from build123d import *

# Parameters (mm, degrees)
ESBO_O1_W                         = 40
ESBO_O1_H                         = 15
RESSALTO_EXTRUS_O1_DEPTH          = 3
ESBO_O3_W                         = 40
ESBO_O3_H                         = 15
RESSALTO_EXTRUS_O2_DEPTH          = 2
CORTE_EXTRUS_O1_REACH             = 26.418
ESBO_O2_R                         = 2.5
ESBO_O2_R_2                       = 0.75
CORTE_EXTRUS_O1_DIRECTION_2_REACH = 26.418
ESBO_O5_W                         = 20
ESBO_O5_H                         = 15
RESSALTO_EXTRUS_O4_DEPTH          = 60
CHANFRO1_SIZE                     = 19.068057482
CHANFRO1_SIZE_2                   = 16
FILETE4_R                         = 10
ESBO_O6_W                         = 12.577854287
ESBO_O6_H                         = 9
CORTE_EXTRUS_O2_DEPTH             = 81.237970309
FILETE5_R                         = 4.5
CIRPATTERN1_COUNT                 = 2
FILLET1_R                         = 4.5


# Some blends are built 0.0001 mm under size
with BuildPart() as part:
    # Esbo_o1 → Ressalto-extrus_o1 (new body)
    with BuildSketch(Plane.XY):
        with Locations((2.5, 1.5)):
            Rectangle(ESBO_O1_W, ESBO_O1_H)
    extrude(amount=-RESSALTO_EXTRUS_O1_DEPTH)

    # Esbo_o3 → Ressalto-extrus_o2 (add)
    with BuildSketch(Plane.XY):
        with Locations((2.5, 1.5)):
            Rectangle(ESBO_O3_W, ESBO_O3_H)
    extrude(amount=RESSALTO_EXTRUS_O2_DEPTH)

    # Corte-extrus_o1: up to this face of the body (flat: up to its plane)
    corte_extrus_o1_end = Plane(part.part.faces().sort_by_distance((2.5, 1.5, 2))[0])
    # Esbo_o2 → Corte-extrus_o1 (cut, up to the picked face)
    with BuildSketch(Plane.XY, mode=Mode.PRIVATE) as corte_extrus_o1_sk1:
        with Locations(Location((2.5, 1.5, 0), (0, 0, 180))):
            Circle(ESBO_O2_R)
    corte_extrus_o1_tool1 = split(extrude(corte_extrus_o1_sk1.sketch, amount=CORTE_EXTRUS_O1_REACH, mode=Mode.PRIVATE), bisect_by=corte_extrus_o1_end, keep=Keep.BOTH, mode=Mode.PRIVATE)
    # Esbo_o2 → Corte-extrus_o1 (cut, up to the picked face)
    with BuildSketch(Plane.XY, mode=Mode.PRIVATE) as corte_extrus_o1_sk2:
        with Locations(Location((-6, 1.5, 0), (0, 0, 180))):
            Circle(ESBO_O2_R_2)
    corte_extrus_o1_tool2 = split(extrude(corte_extrus_o1_sk2.sketch, amount=CORTE_EXTRUS_O1_REACH, mode=Mode.PRIVATE), bisect_by=corte_extrus_o1_end, keep=Keep.BOTH, mode=Mode.PRIVATE)
    corte_extrus_o1_1 = corte_extrus_o1_tool1.solids().sort_by(Axis((2.5, 1.5, 0), (0, 0, 1)))[0]
    add(corte_extrus_o1_1, mode=Mode.SUBTRACT)
    corte_extrus_o1_2 = corte_extrus_o1_tool2.solids().sort_by(Axis((-6, 1.5, 0), (0, 0, 1)))[0]
    add(corte_extrus_o1_2, mode=Mode.SUBTRACT)
    corte_extrus_o1 = corte_extrus_o1_1 + corte_extrus_o1_2  # Corte-extrus_o1 as one shape, for the pattern or mirror that repeats it

    # Corte-extrus_o1 direction 2: up to this face of the body (flat: up to its plane)
    corte_extrus_o1_direction_2_end = Plane(part.part.faces().sort_by_distance((2.5, 1.5, -3))[0])
    # Esbo_o2 → Corte-extrus_o1 direction 2 (cut, up to the picked face)
    with BuildSketch(Plane.XY, mode=Mode.PRIVATE) as corte_extrus_o1_direction_2_sk1:
        with Locations(Location((2.5, 1.5, 0), (0, 0, 180))):
            Circle(ESBO_O2_R)
    corte_extrus_o1_direction_2_tool1 = split(extrude(corte_extrus_o1_direction_2_sk1.sketch, amount=-CORTE_EXTRUS_O1_DIRECTION_2_REACH, mode=Mode.PRIVATE), bisect_by=corte_extrus_o1_direction_2_end, keep=Keep.BOTH, mode=Mode.PRIVATE)
    # Esbo_o2 → Corte-extrus_o1 direction 2 (cut, up to the picked face)
    with BuildSketch(Plane.XY, mode=Mode.PRIVATE) as corte_extrus_o1_direction_2_sk2:
        with Locations(Location((-6, 1.5, 0), (0, 0, 180))):
            Circle(ESBO_O2_R_2)
    corte_extrus_o1_direction_2_tool2 = split(extrude(corte_extrus_o1_direction_2_sk2.sketch, amount=-CORTE_EXTRUS_O1_DIRECTION_2_REACH, mode=Mode.PRIVATE), bisect_by=corte_extrus_o1_direction_2_end, keep=Keep.BOTH, mode=Mode.PRIVATE)
    corte_extrus_o1_direction_2_1 = corte_extrus_o1_direction_2_tool1.solids().sort_by(Axis((2.5, 1.5, 0), (0, 0, -1)))[0]
    add(corte_extrus_o1_direction_2_1, mode=Mode.SUBTRACT)
    corte_extrus_o1_direction_2_2 = corte_extrus_o1_direction_2_tool2.solids().sort_by(Axis((-6, 1.5, 0), (0, 0, -1)))[0]
    add(corte_extrus_o1_direction_2_2, mode=Mode.SUBTRACT)
    corte_extrus_o1_direction_2 = corte_extrus_o1_direction_2_1 + corte_extrus_o1_direction_2_2  # Corte-extrus_o1 direction 2 as one shape, for the pattern or mirror that repeats it

    # Esbo_o5 → Ressalto-extrus_o4 (add)
    with BuildSketch(Plane.ZY.offset(17.5)):
        with Locations((-0.5, 1.5)):
            Rectangle(ESBO_O5_W, ESBO_O5_H)
    extrude(amount=RESSALTO_EXTRUS_O4_DEPTH)

    # Chanfro1
    # the kernel refuses this chamfer: 19.068057482, 16 mm, written as the material it takes off along each edge
    with BuildSketch(Plane(origin=(-17.5, 58.146127732, -10.5), x_dir=(-0.9996889667359941, 0, -0.024939322090234247), z_dir=(0, -1, 0))) as chanfro1_piece_1_section:
        Polygon((CHANFRO1_SIZE * 0.99968896671, -CHANFRO1_SIZE * 0.0249393220896), (-CHANFRO1_SIZE_2 * 0.0249393220902, -CHANFRO1_SIZE_2 * 0.999688966736), (0, 0), align=None)
    chanfro1_piece_1 = extrude(amount=113.292255464, mode=Mode.PRIVATE)
    chanfro1_piece_1 = split(chanfro1_piece_1, bisect_by=Plane(origin=(-25.155035178, 1.5, -3), z_dir=(0, 0, -1)), keep=Keep.TOP, mode=Mode.PRIVATE)
    add(chanfro1_piece_1, mode=Mode.SUBTRACT)
    with BuildSketch(Plane(origin=(-17.5, 58.146127732, -10.5), x_dir=(-0.9996889667359941, 0, -0.024939322090234247), z_dir=(0, -1, 0))) as chanfro1_piece_2_section:
        Polygon((CHANFRO1_SIZE * 0.99968896671, -CHANFRO1_SIZE * 0.0249393220896), (-CHANFRO1_SIZE_2 * 0.0249393220902, -CHANFRO1_SIZE_2 * 0.999688966736), (0, 0), align=None)
    chanfro1_piece_2 = extrude(amount=113.292255464, mode=Mode.PRIVATE)
    chanfro1_piece_2 = split(chanfro1_piece_2, bisect_by=Plane(origin=(-18.373305927, 1.5, 2), z_dir=(0, 0, 1)), keep=Keep.TOP, mode=Mode.PRIVATE)
    add(chanfro1_piece_2, mode=Mode.SUBTRACT)
    with BuildSketch(Plane(origin=(-17.5, -55.146127732, 9.5), x_dir=(-0.9996889667359941, 0, 0.024939322090234247), z_dir=(0, 1, 0))) as chanfro1_piece_3_section:
        Polygon((CHANFRO1_SIZE * 0.99968896671, -CHANFRO1_SIZE * 0.0249393220896), (-CHANFRO1_SIZE_2 * 0.0249393220902, -CHANFRO1_SIZE_2 * 0.999688966736), (0, 0), align=None)
    chanfro1_piece_3 = extrude(amount=113.292255464, mode=Mode.PRIVATE)
    chanfro1_piece_3 = split(chanfro1_piece_3, bisect_by=Plane(origin=(-25.155035178, 1.5, 2), z_dir=(0, 0, 1)), keep=Keep.TOP, mode=Mode.PRIVATE)
    add(chanfro1_piece_3, mode=Mode.SUBTRACT)
    with BuildSketch(Plane(origin=(-17.5, -55.146127732, 9.5), x_dir=(-0.9996889667359941, 0, 0.024939322090234247), z_dir=(0, 1, 0))) as chanfro1_piece_4_section:
        Polygon((CHANFRO1_SIZE * 0.99968896671, -CHANFRO1_SIZE * 0.0249393220896), (-CHANFRO1_SIZE_2 * 0.0249393220902, -CHANFRO1_SIZE_2 * 0.999688966736), (0, 0), align=None)
    chanfro1_piece_4 = extrude(amount=113.292255464, mode=Mode.PRIVATE)
    chanfro1_piece_4 = split(chanfro1_piece_4, bisect_by=Plane(origin=(-18.373305927, 1.5, -3), z_dir=(0, 0, -1)), keep=Keep.TOP, mode=Mode.PRIVATE)
    add(chanfro1_piece_4, mode=Mode.SUBTRACT)

    # Filete4
    # the kernel refuses this fillet: 10 mm, written as the material it adds along each edge
    with BuildSketch(Plane(origin=(-27.629905537, 9, -3), x_dir=(1, 0, 0), z_dir=(0, -1, 0)), Plane(origin=(-27.629905537, -6, 2), x_dir=(1, 0, 0), z_dir=(0, 1, 0))) as filete4_piece_1:
        with BuildLine():
            CenterArc((FILETE4_R * 0.363970234266, -FILETE4_R), FILETE4_R, 90, 40)
            Line((-FILETE4_R * 0.27881737542, -FILETE4_R * 0.233955556881), (0, 0))
            Line((0, 0), (FILETE4_R * 0.363970234266, 0))
        make_face()
    extrude(amount=15)
    # the kernel refuses this fillet: 10 mm, written as the material it takes off along each edge
    with BuildSketch(Plane(origin=(-77.5, 9, 34.5), x_dir=(0, -1, 0), z_dir=(0, 0, -1))) as filete4_2_piece_1:
        with BuildLine():
            CenterArc((FILETE4_R, -FILETE4_R), FILETE4_R, 90, 90)
            Line((0, -FILETE4_R), (0, 0))
            Line((0, 0), (FILETE4_R, 0))
        make_face()
    extrude(amount=70, mode=Mode.SUBTRACT)
    with BuildSketch(Plane(origin=(-77.5, -6, -35.5), x_dir=(1, 0, 0), z_dir=(0, 0, 1))) as filete4_2_piece_2:
        with BuildLine():
            CenterArc((FILETE4_R, FILETE4_R), FILETE4_R, 180, 90)
            Line((0, FILETE4_R), (0, 0))
            Line((0, 0), (FILETE4_R, 0))
        make_face()
    extrude(amount=70, mode=Mode.SUBTRACT)
    with BuildSketch(Plane(origin=(-36.568057482, 18.099255857, -10.5), x_dir=(0.7660444431190706, 0, 0.6427876096864291), z_dir=(0, -1, 0))) as filete4_2_piece_3:
        with BuildLine():
            CenterArc((FILETE4_R * 0.363970234266, FILETE4_R), FILETE4_R, 230, 40)
            Line((-FILETE4_R * 0.27881737542, FILETE4_R * 0.233955556881), (0, 0))
            Line((0, 0), (FILETE4_R * 0.363970234266, 0))
        make_face()
    extrude(amount=33.198511713, mode=Mode.SUBTRACT)
    with BuildSketch(Plane(origin=(-36.568057482, -15.099255857, 9.5), x_dir=(-1, 0, 0), z_dir=(0, 1, 0))) as filete4_2_piece_4:
        with BuildLine():
            CenterArc((FILETE4_R * 0.363970234266, -FILETE4_R), FILETE4_R, 90, 40)
            Line((-FILETE4_R * 0.27881737542, -FILETE4_R * 0.233955556881), (0, 0))
            Line((0, 0), (FILETE4_R * 0.363970234266, 0))
        make_face()
    extrude(amount=33.198511713, mode=Mode.SUBTRACT)

    # Esbo_o6 → Corte-extrus_o2 (cut, through all)
    with BuildSketch(Plane.XY.offset(9.5)):
        with BuildLine():
            Line((-40.207759824, 6), (-43.207759824, 6))
            Line((-43.207759824, 6), (-67.5, 6))
            ThreePointArc((-67.5, 6), (-71.468626967, 4.766281297), (-74.038348415, 1.5))
            ThreePointArc((-74.038348415, 1.5), (-71.468626967, -1.766281297), (-67.5, -3))
            Line((-67.5, -3), (-43.207759824, -3))
            Line((-43.207759824, -3), (-40.207759824, -3))
            Line((-40.207759824, -3), (-40.207759824, 6))
        make_face()
        with Locations((-33.918832681, 1.5)):
            Rectangle(ESBO_O6_W, ESBO_O6_H)
    extrude(amount=-CORTE_EXTRUS_O2_DEPTH, mode=Mode.SUBTRACT)

    # Filete5
    filete5_edges = [part.edges().sort_by_distance(p)[0] for p in [
        (-27.629905537, -3, -0.5),
        (-27.629905537, 6, -0.5),
        (22.5, -6, -0.5),
        (22.5, 9, -0.5),
    ]]
    fillet(filete5_edges, radius=FILETE5_R - 0.0001)  # a hair under: the kernel refuses the full size

    # CirPattern1: Corte-extrus_o1, Corte-extrus_o1 direction 2 ×2 about axis
    cirpattern1_axis = Axis((2.5, 1.5, 0), (0, 0, 1))
    add([corte_extrus_o1.rotate(cirpattern1_axis, i * 360 / CIRPATTERN1_COUNT) for i in range(1, CIRPATTERN1_COUNT)], mode=Mode.SUBTRACT)
    add([corte_extrus_o1_direction_2.rotate(cirpattern1_axis, i * 360 / CIRPATTERN1_COUNT) for i in range(1, CIRPATTERN1_COUNT)], mode=Mode.SUBTRACT)

    # Fillet1
    # the kernel refuses this fillet: 4.5 mm, written as the material it adds along each edge
    with BuildSketch(Plane(origin=(-74.038348415, 1.5, 9.5), x_dir=(0.8237540050665563, -0.566947386568461, 0), z_dir=(0, 0, -1))) as fillet1_piece_1:
        with BuildLine():
            CenterArc((5.385987308, -3.706897217), FILLET1_R, 55.462463306, 179.999811631)
            ThreePointArc((2.834717975, -7.413786046), (0.265006635, -4.147503786), (0, 0))
            ThreePointArc((0, 0), (3.968622227, 1.233715441), (7.937244454, 0))
        make_face()
    extrude(amount=20)
    # the kernel refuses this fillet: 4.5 mm, written as the material it takes off along each edge
    with BuildSketch(Plane(origin=(-77.182458366, 1.5, -15.968577797), x_dir=(0.3543987879296305, 0.9350943797895531, 0), z_dir=(0, 0, 1))) as fillet1_2_piece_1:
        with BuildLine():
            CenterArc((1.695259117, -4.473004216), FILLET1_R, 83.720910198, 54.071383579)
            ThreePointArc((-1.63795498, -1.449813223), (-0.858738838, -0.679985448), (0, 0))
            ThreePointArc((0, 0), (1.093715559, 0.05999063), (2.187431119, 0))
        make_face()
    extrude(amount=30.937155594, mode=Mode.SUBTRACT)


with BuildPart() as part_1:
    # Body-Move_Copy2: moved
    add(part.part.moved(Location((0, 0, 1))))


solid = part_1.part
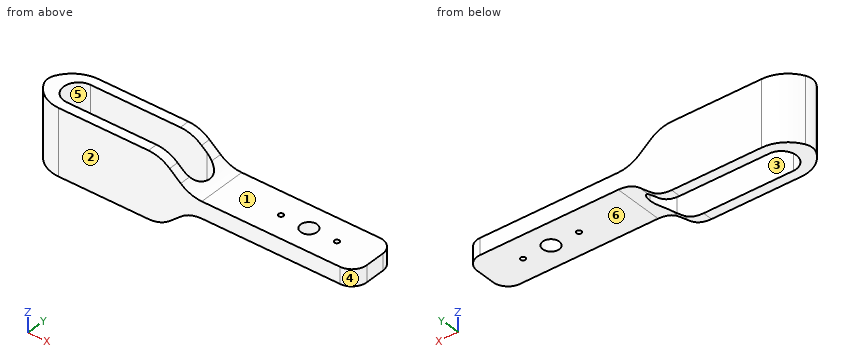
Part model, mm, in its own coordinate system. Face numbers are marked on the shaded views. A direction names the side the tool comes from. Round coordinates to 2 decimals unless told otherwise and drop trailing zeros. Order: outer loops, then holes, each group sorted by start corner. A loop starts at its lowest first (then second) coordinate and runs counter-clockwise, first axis right, second up. Notation, with made-up numbers: (-25, 1.25) -> (-5, 1.25) arc R21 cw to (-5, 38.25) -> close; hole circle Ø3 at (5, -9). An arc over 180 degrees is marked (long way). Put each result on its own line as item: value.
Q1. Band-saw the part on C-C (x = -47). Give the cut face in (y, z).
From the geometry:
outline: (-6, -9.5) -> (-3, -9.5) -> (-3, 10.5) -> (-6, 10.5) -> close; (6, -9.5) -> (9, -9.5) -> (9, 10.5) -> (6, 10.5) -> close
Q2. Tool access for the marked faces 4, 5 and 6: list every direction of +Z, -Z, +X, -X, +Y, -Y with a clear straight run to the whole face (end or side of a thin tool).
From the geometry:
face 4: +Z, -Z, +X, -Y
face 5: +Z, -Z
face 6: -Z, +X, +Y, -Y
Q3. Pin check, flat tips, straight feed: pin 1 Ø4 at (x, y) = (-11.5, 6.5) entering from +Z; pin 2 Ø1.7 at (x, y) = (11, 1.5) entering from -Z; pin 3 Ø5 at (x, z) = (-24.5, -6) entering from +Y; pin 4 Ø6 at (y, z) = (4.5, 2.5) entering from -X. Stop position of each tip, or through.
From the geometry:
pin 1: stops at z = 3
pin 2: stops at z = -2
pin 3: passes through
pin 4: stops at x = -76.9
Q4. Pull direction Y, two halves, no side cores. Call the marked faces 1, 2 and 3: pulls with the +Y half, pulls with the -Y half, needs draft (parallel to the pull), parting line crosses it, or undercut.
From the geometry:
face 1: needs draft
face 2: pulls with the -Y half
face 3: undercut
Q5. Wall check: line 1 (Y direction, x = -6, z = 0.5); line 2 (Y direction, x = -54.5, z = -4.5); line 3 (Z direction, x = -20, y = -3.5). Give the ranges that are in metal, low to high. Write a range as [from, to].
From the geometry:
line 1: y = [-6, 0.75], [2.25, 9]
line 2: y = [-6, -3], [6, 9]
line 3: z = [-2, 3]
Q6. Band-saw the part on B-B (x = 2.5). Give the cut face in (y, z), and give its area (3 significant figures).
From the geometry:
outline: (-6, -2) -> (-1, -2) -> (-1, 3) -> (-6, 3) -> close; (4, -2) -> (9, -2) -> (9, 3) -> (4, 3) -> close
area: 50.0 mm2
Q7. Band-saw the part on D-D (x = -16). Give the cut face in (y, z), and give its area (3 significant figures).
From the geometry:
outline: (-6, -2) -> (9, -2) -> (9, 3) -> (-6, 3) -> close
area: 75.0 mm2
Q8. Band-saw the part on A-A (z = 1.25). State how many separate pieces and enclosed holes the cut face has, and give its area (3 significant figures).
From the geometry:
separate pieces: 1
enclosed holes: 4
area: 1,040 mm2
